from build123d import *

# Parameters (mm, degrees)
F1_DEPTH    = 4
F3_DEPTH    = 4
F4_T1_DEPTH = 8.9373301178
F4_T3_DEPTH = 5.4979166118


# Not quite as in the source:
# - a fillet or chamfer that OpenCascade refuses, or shapes differently, is made with other operations: its cross-section is extruded or revolved along the edge and cut away or added


with BuildPart() as f1:
    # F0 (on Top) → F1 (new body)
    with BuildSketch(Plane.XY):
        with BuildLine():
            Line((5.4043182717, 11.9166336954), (9.2633608729, 11.9166336954))
            Line((9.2633608729, 11.9166336954), (13.1224034741, 11.9166336954))
            ThreePointArc((13.1224034741, 11.9166336954), (12.5478266836, 12.1546311946), (12.3098291843, 12.7292079851))
            Line((12.3098291843, 12.7292079851), (12.3098291843, 17.1262745588))
            ThreePointArc((12.3098291843, 17.1262745588), (12.1943632439, 17.8955690891), (11.8581410497, 18.5970682651))
            ThreePointArc((11.8581410497, 18.5970682651), (13.7265197912, 18.7234015951), (15.3986439109, 19.5664912462))
            ThreePointArc((15.3986439109, 19.5664912462), (17.0218223076, 21.5886397467), (17.5903830677, 24.1185668856))
            ThreePointArc((17.5903830677, 24.1185668856), (17.2823984437, 26.1835910199), (16.4102166891, 28.0805565417))
            ThreePointArc((16.4102166891, 28.0805565417), (16.638828313, 29.724361375), (16.4102166891, 31.3681662083))
            ThreePointArc((16.4102166891, 31.3681662083), (14.3575671426, 31.3236587754), (12.6471198819, 30.1879998296))
            ThreePointArc((12.6471198819, 30.1879998296), (10.9641887914, 30.4698973914), (9.2633608729, 30.6074026007))
            ThreePointArc((9.2633608729, 30.6074026007), (7.5625329544, 30.4698973914), (5.8796018638, 30.1879998296))
            ThreePointArc((5.8796018638, 30.1879998296), (4.1691546032, 31.3236587754), (2.1165050566, 31.3681662083))
            ThreePointArc((2.1165050566, 31.3681662083), (1.8878934327, 29.724361375), (2.1165050566, 28.0805565417))
            ThreePointArc((2.1165050566, 28.0805565417), (1.244323302, 26.1835910199), (0.936338678, 24.1185668856))
            ThreePointArc((0.936338678, 24.1185668856), (1.5048994381, 21.5886397467), (3.1280778348, 19.5664912462))
            ThreePointArc((3.1280778348, 19.5664912462), (4.8002019546, 18.7234015951), (6.668580696, 18.5970682651))
            ThreePointArc((6.668580696, 18.5970682651), (6.3323585018, 17.8955690891), (6.2168925614, 17.1262745588))
            Line((6.2168925614, 17.1262745588), (6.2168925614, 12.7292079851))
            ThreePointArc((6.2168925614, 12.7292079851), (5.9788950622, 12.1546311946), (5.4043182717, 11.9166336954))
        make_face()
    extrude(amount=F1_DEPTH)

    # F2 (on Top) → F3 (join, through all)
    with BuildSketch(Plane.XY):
        with BuildLine():
            ThreePointArc((6.2168925614, 16.8439224371), (5.6798309181, 16.5586654348), (5.0929421559, 16.3993909955))
            ThreePointArc((5.0929421559, 16.3993909955), (4.1545493311, 16.4529754412), (3.3199274912, 16.8852470815))
            ThreePointArc((3.3199274912, 16.8852470815), (2.3265556072, 17.5975106191), (1.2477898737, 18.1722901762))
            ThreePointArc((1.2477898737, 18.1722901762), (0.8448717213, 18.2802980548), (0.441953569, 18.1722901762))
            ThreePointArc((0.441953569, 18.1722901762), (0.5289468082, 17.7574058892), (0.8448717213, 17.4747608034))
            ThreePointArc((0.8448717213, 17.4747608034), (1.7862867621, 16.9138981945), (2.5603426512, 16.1382264689))
            ThreePointArc((2.5603426512, 16.1382264689), (3.5961993789, 15.3105799436), (4.8955686661, 15.0466909773))
            ThreePointArc((4.8955686661, 15.0466909773), (5.5689958467, 15.1314623043), (6.2168925614, 15.3337497048))
            Line((6.2168925614, 15.3337497048), (6.2168925614, 16.8439224371))
        make_face()
    extrude(amount=F3_DEPTH)

    # F4: fillet of radius 0.3 on 3 edges, made by hand

    # F4_s2 → F4_t1 (cut)
    with BuildSketch(Plane.XY.offset(-2.4686650589)):
        with BuildLine():
            ThreePointArc((12.1349374505, 11.9166336954), (12.3913198946, 12.0608516606), (12.4012026427, 12.3548467462))
            ThreePointArc((12.4012026427, 12.3548467462), (12.7004552198, 12.0347753771), (13.1224034741, 11.9166336954))
            Line((13.1224034741, 11.9166336954), (12.1349374505, 11.9166336954))
        make_face()
        with BuildLine():
            ThreePointArc((6.1255191031, 12.3548467462), (6.1354018511, 12.0608516606), (6.3917842952, 11.9166336954))
            Line((6.3917842952, 11.9166336954), (5.4043182717, 11.9166336954))
            ThreePointArc((5.4043182717, 11.9166336954), (5.8262665259, 12.0347753771), (6.1255191031, 12.3548467462))
        make_face()
    extrude(amount=F4_T1_DEPTH, mode=Mode.SUBTRACT)

    # F4_s4 → F4_t3 (cut)
    with BuildSketch(Plane.XY.offset(-0.7489583059)):
        with BuildLine():
            ThreePointArc((0.7077089455, 18.2685344716), (0.5003837706, 18.1253146023), (0.4753670818, 17.8745760445))
            ThreePointArc((0.4753670818, 17.8745760445), (0.4420534576, 18.0215692627), (0.441953569, 18.1722901762))
            ThreePointArc((0.441953569, 18.1722901762), (0.5705770014, 18.2321594237), (0.7077089455, 18.2685344716))
        make_face()
    extrude(amount=F4_T3_DEPTH, mode=Mode.SUBTRACT)


solid = f1.part
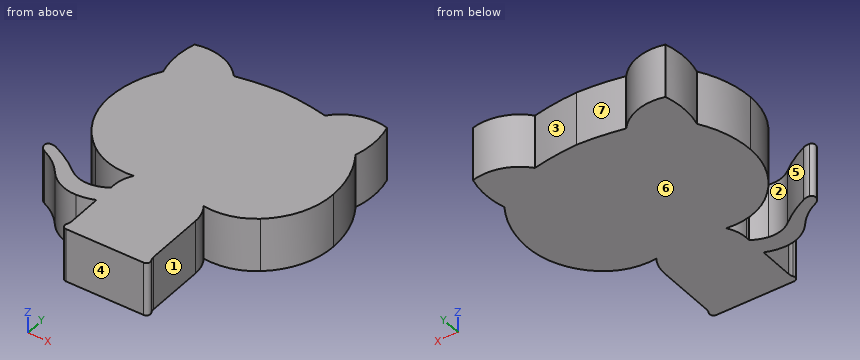
Here's how the part is built. I have some questions about the finished solid (model axes, mm). Face numbers are marked on the shaded views. A direction names the side the tool comes from. Give positions to 0.01 mm unless a question says otherwise; leave off trailing zeros. Order: outer loops, then holes, each group sorted by start corner. A loop starts at its lowest first (then second) coordinate and runs counter-clockwise, first axis right, second up. Notation, with made-up numbers: M 63.25,84.25 L 69.25,84.25 A22 cw 69.25,121.25 Z; hole C 2,-4 d7. An arc over 180 degrees is marked long. Answer as a JSON object with one key per item and string values. Group by question number.
1) On a 3-axis mill with a long thin cutter (end or side, diameter ignored), from which of +Z, -Z, +X, -X, +Y, -Y can I reach the whole of each face in a straight line? I mean the marked faces 5, 6 and 7. Say none if no direction works.
2) I'm going to push flat-ended pins straight in: pin 1 Ø1.5 at (x, z) = (13.5, 2.5) entering from +Y; pin 2 Ø1.5 at (x, z) = (14.5, 2) entering from -Y; pin 3 Ø1.2 at (y, z) = (15, 1) entering from +X. Where does each tip first touch, or does it pass through?
3) Suppose I cut it at B-B, the plane x = 4.5. Write out the boundary of the cut face in (y, z).
4) Suppose I cut it at C-C, the plane y = 27.75. Write out the boundary of the cut face in (x, z).
5) We'd pull the mould along Y, two halves only. Please class the marked faces 1, 2, 3 and 4: pulls with the +Y half, pulls with the -Y half, needs draft (parallel to the pull), parting line crosses it, or undercut.
6) Suppose I cut it at D-D, the plane x = 13.5. Write out the boundary of the cut face in (y, z), plus the area to 3 significant figures.
7) Please list where these lines run through material, in increasing order: L1, parallel to X at y = 13, z = 1.9; L2, parallel to Y at x = 6.5, z = 0.85; L3, parallel to Y at x = 6, z = 0.25. Write a range as [from, to].
Results found:
{
 "1": {"face 5": "+Z, -Z", "face 6": "-Z, +X, -X, +Y, -Y", "face 7": "+Z, -Z, +Y"},
 "2": {"pin 1": "y = 31.29", "pin 2": "y = 18.73", "pin 3": "x = 12.31"},
 "3": {"outline": "M 15.06,0 L 16.39,0 L 16.39,4 L 15.06,4 Z; M 18.82,0 L 31.2,0 L 31.2,4 L 18.82,4 Z"},
 "4": {"outline": "M 1.92,0 L 16.61,0 L 16.61,4 L 1.92,4 Z"},
 "5": {"face 1": "undercut", "face 2": "undercut", "face 3": "pulls with the +Y half", "face 4": "pulls with the -Y half"},
 "6": {"outline": "M 18.67,0 L 30.93,0 L 30.93,4 L 18.67,4 Z", "area": "49.0 mm²"},
 "7": {"L1": "[6.22, 12.31]", "L2": "[11.92, 18.31], [18.58, 30.31]", "L3": "[15.25, 16.71], [18.56, 30.21]"}
}
